The model under review builds one solid part; all positions refer to its coordinate system, in mm. A direction names the side the tool comes from. Coordinates: 2 decimals unless noted, no trailing zeros. Write each loop counter-clockwise with the first axis right and the second up, starting at its lowest first coordinate (ties: lowest second). Pieces come first, ordered by that corner, then holes.
1) Add section B-B, the plane x = 0. State the section outline as (y, z) points, then the cut area to 3 significant figures.
2) Add section D-D, the plane y = -24.5. Give the number of separate pieces and of enclosed holes in the cut face, then the cut area to 3 significant figures.
3) Add section A-A, the plane y = 0. State the section outline as (x, z) points, then the cut area to 3 significant figures.
4) Machinability: for faces 1 (the flat face through (24, -28, 1)), 2 (the flat face through (-24, -28, 1)), 3 (the cylindrical face through (36, -24.4, 6.5)), which of the approach directions +Z, -Z, +X, -X, +Y, -Y give a long, thin tool a straight path to every point of the face, cutting with its end or side? Answer none if there is none.
5) For P1, Ø7, axis at x = 0, y = -36, coming from the +Z side; P2, Ø1, axis at y = -32.5, z = 1.5, coming from the +X side; P3, Ø0.6, axis at x = -24.5, z = 1.5, coming from the -Y side, all flat-tipped, find the tip position at first contact; note any pin that passes through.
6) Mouldability with a two-part tool opening along X and no side actions: class faces 4 (the flat face through (-18, -23, 10)), 5 (the cylindrical face through (-20.11, 25.51, 4.93)), 6 (the cylindrical face through (41.9, -27.43, 1.49)) as released by +X, released by -X, zero draft, split by the parting line, or undercut.
7) For line 1 (Y direction, x = -19, z = 6.5); line 2 (Y direction, x = 0, z = 0.85); line 3 (Z direction, x = 19, y = 11.5), list the stretches that pass through material, from the lowest coordinate up.
8) Add section C-C, the plane z = 6. State the section outline as (x, y) points.
from build123d import *

# Parameters (mm, degrees)
F0_R     = 3
F0_R_2   = 3.05
F0_R_3   = 1.5
F1_DEPTH = 3
F2_DEPTH = 10
F3_R     = 0.49999


# Not quite as in the source:
# - a fillet or chamfer is up to 0.001 mm smaller than in the source, because OpenCascade refuses the exact size
# - a feature names something its author has since deleted; it is built from what else it names


with BuildPart() as f1:
    # F0 (on Top) → F1 (new body)
    with BuildSketch(Plane.XY):
        with BuildLine():
            ThreePointArc((42.5, 26), (41.9142135624, 27.4142135624), (40.5, 28))
            Line((40.5, 28), (-40.5, 28))
            ThreePointArc((-40.5, 28), (-41.9142135624, 27.4142135624), (-42.5, 26))
            Line((-42.5, 26), (-42.5, -26))
            ThreePointArc((-42.5, -26), (-41.9142135624, -27.4142135624), (-40.5, -28))
            Line((-40.5, -28), (-7, -28))
            ThreePointArc((-7, -28), (-5.5857864376, -28.5857864376), (-5, -30))
            Line((-5, -30), (-5, -36))
            ThreePointArc((-5, -36), (0, -41), (5, -36))
            Line((5, -36), (5, -30))
            ThreePointArc((5, -30), (5.5857864376, -28.5857864376), (7, -28))
            Line((7, -28), (40.5, -28))
            ThreePointArc((40.5, -28), (41.9142135624, -27.4142135624), (42.5, -26))
            Line((42.5, -26), (42.5, 26))
        make_face()
        with Locations((-19, -24.5)):
            Circle(F0_R, mode=Mode.SUBTRACT)
        with Locations((0, -36)):
            Circle(F0_R_2, mode=Mode.SUBTRACT)
        with Locations((39, -24.5)):
            Circle(F0_R, mode=Mode.SUBTRACT)
        with Locations((-19, 24.5)):
            Circle(F0_R, mode=Mode.SUBTRACT)
        Circle(F0_R_3, mode=Mode.SUBTRACT)
        with Locations((39, 24.5)):
            Circle(F0_R, mode=Mode.SUBTRACT)
    extrude(amount=F1_DEPTH)

    # F0 (on Top) → F2 (join)
    with BuildSketch(Plane.XY):
        with Locations((-19, -24.5)):
            Circle(F0_R)
        with Locations((-19, -24.5)):
            Circle(F0_R_3, mode=Mode.SUBTRACT)
        with Locations((-19, 24.5)):
            Circle(F0_R)
        with Locations((-19, 24.5)):
            Circle(F0_R_3, mode=Mode.SUBTRACT)
        with Locations((39, 24.5)):
            Circle(F0_R)
        with Locations((39, 24.5)):
            Circle(F0_R_3, mode=Mode.SUBTRACT)
        with Locations((39, -24.5)):
            Circle(F0_R)
        with Locations((39, -24.5)):
            Circle(F0_R_3, mode=Mode.SUBTRACT)
    extrude(amount=F2_DEPTH)

    # F3 (radius 0.5 in the source; OpenCascade refuses exactly that, so slightly less here)
    f3_edges = [f1.edges().sort_by_distance(p)[0] for p in [
        (23.75, -28, 3),
        (23.75, -28, 0),
    ]]
    fillet(f3_edges, radius=F3_R)


solid = f1.part
Geometry results:
1. outline: (-41, 0.5) arc R0.5 ccw to (-40.5, 0) - (-39.05, 0) - (-39.05, 3) - (-40.5, 3) arc R0.5 ccw to (-41, 2.5) - close; (-32.95, 0) - (-1.5, 0) - (-1.5, 3) - (-32.95, 3) - close; (1.5, 0) - (27.5, 0) arc R0.5 ccw to (28, 0.5) - (28, 2.5) arc R0.5 ccw to (27.5, 3) - (1.5, 3) - close
1. area: 179 mm2
2. separate pieces: 3
2. enclosed holes: 0
2. area: 279 mm2
3. outline: (-42.5, 0.5) arc R0.5 ccw to (-42, 0) - (-1.5, 0) - (-1.5, 3) - (-42, 3) arc R0.5 ccw to (-42.5, 2.5) - close; (1.5, 0) - (42, 0) arc R0.5 ccw to (42.5, 0.5) - (42.5, 2.5) arc R0.5 ccw to (42, 3) - (1.5, 3) - close
3. area: 246 mm2
4. face 1: +Z, -Z, +X, -Y
4. face 2: +Z, -Z, -X, -Y
4. face 3: +Z
5. P1: stops at z = 3
5. P2: stops at x = 5
5. P3: stops at y = -28
6. face 4: zero draft
6. face 5: undercut
6. face 6: released by +X
7. line 1: y = -27.5 to -26, -23 to -21.5, 21.5 to 23, 26 to 27.5
7. line 2: y = -41 to -39.05, -32.95 to -1.5, 1.5 to 28
7. line 3: z = 0 to 3
8. outline: circle Ø6 at (-19, -24.5); circle Ø6 at (-19, 24.5); circle Ø6 at (39, -24.5); circle Ø6 at (39, 24.5); hole circle Ø3 at (-19, -24.5); hole circle Ø3 at (-19, 24.5); hole circle Ø3 at (39, -24.5); hole circle Ø3 at (39, 24.5)
